```python
from build123d import *

# Parameters (mm, degrees)
BOSS_EXTRUDE1_DEPTH = 10
SKETCH2_R           = 2.5
CUT_EXTRUDE1_DEPTH  = 88.866025
SKETCH3_R           = 2.5
CUT_EXTRUDE2_DEPTH  = 6


with BuildPart() as part:
    # Sketch1 → Boss-Extrude1 (new body)
    with BuildSketch(Plane(origin=(0, 0, 0), x_dir=(1, 0, 0), z_dir=(0, 1, 0))):
        Polygon((-3, 71.01408311), (-41, 5.196152423), (-46.196152423, 2.196152423), (-43.196152423, -3), (-38, 0), (38, 0), (43.196152423, -3), (46.196152423, 2.196152423), (41, 5.196152423), (3, 71.01408311), (3, 77.01408311), (-3, 77.01408311), align=None)
    extrude(amount=BOSS_EXTRUDE1_DEPTH)

    # Sketch2 → Cut-Extrude1 (cut)
    with BuildSketch(Plane(origin=(-9.5, 0, -16.454482672), x_dir=(0.866025404, 0, -0.5), z_dir=(0.5, 0, 0.866025404))):
        with Locations((-35.908965344, 5)):
            Circle(SKETCH2_R)
    cut_extrude1 = extrude(amount=-CUT_EXTRUDE1_DEPTH, mode=Mode.SUBTRACT)

    # Mirror6: Cut-Extrude1 across plane
    add(cut_extrude1.mirror(Plane.ZY), mode=Mode.SUBTRACT)

    # Sketch3 → Cut-Extrude2 (cut)
    with BuildSketch(Plane.ZY.offset(3)):
        with Locations((-74.01408311, 5)):
            Circle(SKETCH3_R)
    extrude(amount=-CUT_EXTRUDE2_DEPTH, mode=Mode.SUBTRACT)


solid = part.part
```
Geometry: final body of the model. Coordinates: model frame, mm. A direction names the side the tool comes from. Round coordinates to 2 decimals unless told otherwise and drop trailing zeros. Write each loop counter-clockwise with the first axis right and the second up, starting at its lowest first coordinate (ties: lowest second). Pieces come first, ordered by that corner, then holes.
Item 1: Mould query, pull axis Y, two halves, no side actions, for faces 1 (the face through (-0.04, 5.75, -71.63)), 2 (the face through (-3, 2.7, -75.4)), 3 (the face through (-40.01, 5.75, -2.25)), 4 (the face through (-1, 10, -29)). Classes: +Y half, -Y half, draft (parallel to the pull), parting line (faces both ways), or undercut.
Item 2: Section query A-A (y = 5). Return loops of the section in (x, z), plus the area to 3 significant figures.
Item 3: Section query B-B (z = -54). Return loops of the section in (x, y).
Item 4: Material intervals for L1, parallel to X at y = 9.25, z = -72.5; L2, parallel to Z at x = 32, y = 7.5; L3, parallel to Z at x = 16.5, y = 0.75, sorted ascending.
Item 5: Pin query (flat end, axial travel): P1, Ø3, axis at x = 1.5, y = 7.5, coming from the +Z side; P2, Ø6, axis at y = 2.5, z = -49, coming from the -X side; P3, Ø6, axis at y = 6, z = -25, coming from the -X side. Return the tip coordinate at first contact, or that it passes through.
Item 6: Section query C-C (x = 28). Return loops of the section in (y, z).
Item 7: Set-up query: faces 5 (the face through (40.01, 5.75, -2.25)), 6 (the face through (3, 2.7, -72.6)), 7 (the face through (39.407, 2.708, 0.812)). Return all of +Z, -Z, +X, -X, +Y, -Y with unobstructed straight access to the full face (end or side cutting, diameter ignored); none if empty.
Completed:
1. face 1: undercut
1. face 2: draft
1. face 3: undercut
1. face 4: +Y half
2. outline: (-46.2, -2.2) - (-45.76, -2.45) - (-42.76, 2.75) - (-43.2, 3) - close; (-41.43, -4.95) - (-41, -5.2) - (-3, -71.01) - (-3, -71.51) - (3, -71.51) - (3, -71.01) - (41, -5.2) - (41.43, -4.95) - (38.43, 0.25) - (38, 0) - (-38, 0) - (-38.43, 0.25) - close; (-3, -77.01) - (3, -77.01) - (3, -76.51) - (-3, -76.51) - close; (42.76, 2.75) - (45.76, -2.45) - (46.2, -2.2) - (43.2, 3) - close
2. area: 3,320 mm2
3. outline: (-12.82, 0) - (12.82, 0) - (12.82, 10) - (-12.82, 10) - close
4. L1: x = -3 to 3
4. L2: z = -20.78 to 0
4. L3: z = -47.63 to 0
5. P1: stops at z = 0
5. P2: stops at x = -17.44
5. P3: stops at x = -31.3
6. outline: (0, -27.71) - (10, -27.71) - (10, 0) - (0, 0) - close
7. face 5: none
7. face 6: -Z, +X, +Y, -Y
7. face 7: +Z, +Y, -Y
